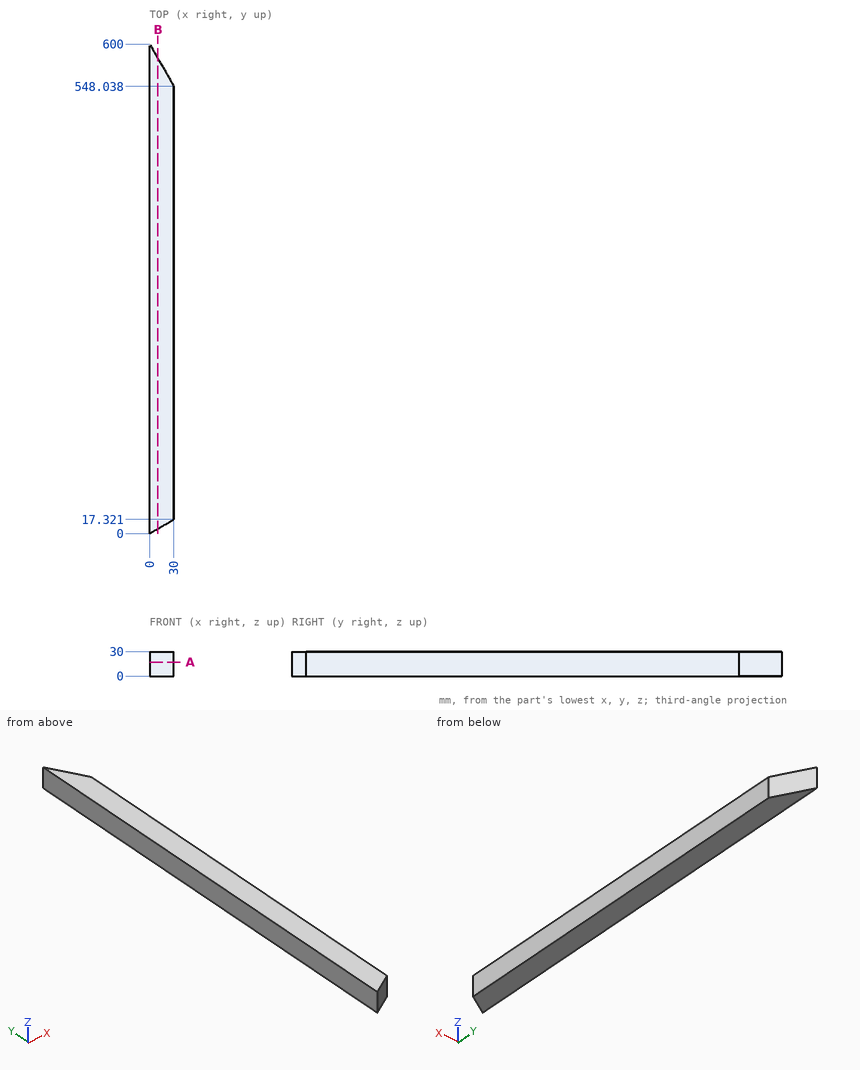
Print and shaded views of the part. All mm, measured from the part's lowest x, y and z. Give positions to 0.01 mm unless a question says otherwise; leave off trailing zeros. Loops run counter-clockwise (first coordinate to the right, second up) from the corner with the lowest first, then second, coordinate; pieces in that order, holes last. Notation, with made-up numbers: (48.25, 48.5) - (88.25, 48.5) arc R19 ccw to (88.25, 64.5) - close; hole circle Ø7 at (55.25, -2). An arc over 180 degrees is marked (long way). Use a Markdown table: item, result.
(1) Band-saw the part on A-A (z = 17). Give the cut face in (x, y).
Taken from the geometry:
| item | result |
|---|---|
| outline | (0, 0) - (30, 17.32) - (30, 548.04) - (0, 600) - close |
(2) Drop a flat-ended pin along its axis: pin 1 Ø4 at (x, z) = (6, 21) entering from +Y. Give the stop position or say it passes through.
Taken from the geometry:
| item | result |
|---|---|
| pin 1 | y = 593.07 |
(3) Wall check: line 1 along Y through (x, z) = (26.25, 3) (1 decimal); line 2 along Y through (x, z) = (18.5, 3.5) (1 decimal); line 3 along X through (y, z) = (559, 21.75). Give the ranges that are in metal, low to high.
Taken from the geometry:
| item | result |
|---|---|
| line 1 | 15.2 to 554.5 |
| line 2 | 10.7 to 568 |
| line 3 | 0 to 23.67 |
(4) Band-saw the part on B-B (x = 10.25). Give the cut face in (y, z), and give its area (3 significant figures).
Taken from the geometry:
| item | result |
|---|---|
| outline | (5.92, 0) - (582.25, 0) - (582.25, 30) - (5.92, 30) - close |
| area | 17,300 mm2 |
